CAD build for the part. Positions are in the model's coordinates, mm. A direction names the side the tool comes from. Give positions to 0.01 mm unless a question says otherwise; leave off trailing zeros. Write each loop counter-clockwise with the first axis right and the second up, starting at its lowest first coordinate (ties: lowest second). Pieces come first, ordered by that corner, then holes. Notation, with made-up numbers: (25.25, 55) - (73.25, 55) arc R21 ccw to (73.25, 62) - close; hole circle Ø5 at (51, 0.5). An arc over 180 degrees is marked (long way). Answer as a JSON object with one key per item and string values.
from build123d import *

# Parameters (mm, degrees)
BOSS_EXTRUDE1_DEPTH = 50.8
SKETCH2_W           = 11.43
SKETCH2_H           = 24.13
BOSS_EXTRUDE2_DEPTH = 25.4
FILLET3_R           = 2.54
SKETCH3_R           = 3.175
CUT_EXTRUDE1_DEPTH  = 199.372898559
SKETCH4_W           = 25.146
SKETCH4_H           = 13.208
SKETCH4_W_2         = 25.908
SKETCH4_H_2         = 8.89
CUT_EXTRUDE2_DEPTH  = 25.4
CHAMFER1_SIZE       = 8.89
SKETCH5_R           = 3.175
CUT_EXTRUDE3_DEPTH  = 202.317710741
SKETCH7_W           = 50.8
SKETCH7_H           = 50.8
BOSS_EXTRUDE4_DEPTH = 6.35
FILLET4_R           = 12.7


with BuildPart() as part:
    # Sketch1 → Boss-Extrude1 (new body)
    with BuildSketch(Plane(origin=(0, 0, 0), x_dir=(1, 0, 0), z_dir=(0, 1, 0))):
        Polygon((-59.171267606, -17.601126761), (-59.171267606, 185.598873239), (42.428732394, 185.598873239), (42.428732394, -17.601126761), (17.028732394, -17.601126761), (17.028732394, 160.198873239), (-33.771267606, 160.198873239), (-33.771267606, -17.601126761), align=None)
    extrude(amount=BOSS_EXTRUDE1_DEPTH)

    # Sketch2 → Boss-Extrude2 (add)
    with BuildSketch(Plane.XY.offset(17.601126761)):
        with Locations((-46.471267606, 25.4)):
            Rectangle(SKETCH2_W, SKETCH2_H)
        with Locations((29.728732394, 25.4)):
            Rectangle(SKETCH2_W, SKETCH2_H)
    extrude(amount=BOSS_EXTRUDE2_DEPTH)

    # Fillet3
    fillet3_edges = [part.edges().sort_by_distance(p)[0] for p in [
        (-46.471267606, 37.465, 17.601126761),
        (-46.471267606, 13.335, 17.601126761),
        (29.728732394, 37.465, 17.601126761),
        (29.728732394, 13.335, 17.601126761),
    ]]
    fillet(fillet3_edges, radius=FILLET3_R)

    # Sketch3 → Cut-Extrude1 (cut, through all)
    with BuildSketch(Plane(origin=(0, 37.465, 0), x_dir=(1, 0, 0), z_dir=(0, 1, 0))):
        with Locations(Location((-47.106267606, -30.301126761, 0), (0, 0, 270))):
            Circle(SKETCH3_R)
        with Locations(Location((29.093732394, -30.301126761, 0), (0, 0, 270))):
            Circle(SKETCH3_R)
    extrude(amount=-CUT_EXTRUDE1_DEPTH, mode=Mode.SUBTRACT)

    # Sketch4 → Cut-Extrude2 (cut)
    with BuildSketch(Plane(origin=(0, 0, -185.598873239), x_dir=(-1, 0, 0), z_dir=(0, 0, -1))):
        with Locations((-17.155732394, 25.4)):
            Rectangle(SKETCH4_W, SKETCH4_H)
        with Locations((8.371267606, 25.4)):
            Rectangle(SKETCH4_W_2, SKETCH4_H)
        with Locations((8.371267606, 36.449)):
            Rectangle(SKETCH4_W_2, SKETCH4_H_2)
        with Locations((33.898267606, 25.4)):
            Rectangle(SKETCH4_W, SKETCH4_H)
        with Locations((8.371267606, 14.351)):
            Rectangle(SKETCH4_W_2, SKETCH4_H_2)
    extrude(amount=-CUT_EXTRUDE2_DEPTH, mode=Mode.SUBTRACT)

    # Chamfer1
    chamfer1_edges = [part.edges().sort_by_distance(p)[0] for p in [
        (-21.325267606, 32.004, -172.898873239),
        (-21.325267606, 18.796, -172.898873239),
        (4.582732394, 18.796, -172.898873239),
        (4.582732394, 32.004, -172.898873239),
    ]]
    chamfer(chamfer1_edges, length=CHAMFER1_SIZE - 0.0001)  # a hair under: the kernel refuses the full size

    # Sketch5 → Cut-Extrude3 (cut, through all)
    with BuildSketch(Plane.XZ):
        with Locations(Location((-8.371267606, -172.898873239, 0), (0, 0, 270))):
            Circle(SKETCH5_R)
    extrude(amount=-CUT_EXTRUDE3_DEPTH, mode=Mode.SUBTRACT)

    # Sketch7 → Boss-Extrude4 (add)
    with BuildSketch(Plane.XY.offset(-160.198873239)):
        with Locations((-8.371267606, 25.4)):
            Rectangle(SKETCH7_W, SKETCH7_H)
    extrude(amount=BOSS_EXTRUDE4_DEPTH)

    # Fillet4
    fillet4_edges = [part.edges().sort_by_distance(p)[0] for p in [
        (-33.771267606, 25.4, -153.848873239),
        (17.028732394, 25.4, -153.848873239),
    ]]
    fillet(fillet4_edges, radius=FILLET4_R)


solid = part.part
Item 1: Mould opens along X. For faces 4 (the flat face through (-59.171, 25, -83)), 5 (the flat face through (-9, 26, -160.199)), 6 (the flat face through (35.444, 25, 30)), 7 (the flat face through (-43, 50.8, -108)) say: +X half, -X half, draft (parallel to the pull), parting line (faces both ways), or undercut.
Entries:
{"face 4": "-X half", "face 5": "undercut", "face 6": "+X half", "face 7": "draft"}
Item 2: Flat gauge pins, fed straight in: P1, Ø7.5, axis at y = 23.5, z = 26, coming from the -X side; P2, Ø5.5, axis at x = 30.5, z = 28, coming from the +Y side (3 decimals); P3, Ø1.5, axis at x = 9, y = 27, coming from the +Z side. Where does each tip first touch, or does it go through?
Entries:
{"P1": "x = -52.19", "P2": "y = 37.465", "P3": "z = -152.63"}
Item 3: Cut at D-D (y = 45.5). Give the cut face in (x, z) (3 decimals).
Entries:
{"outline": "(-59.171, -185.599) - (42.429, -185.599) - (42.429, 17.601) - (17.029, 17.601) - (17.029, -141.149) arc R12.7 cw to (4.329, -153.849) - (-21.071, -153.849) arc R12.7 cw to (-33.771, -141.149) - (-33.771, 17.601) - (-59.171, 17.601) - close; hole circle Ø6.35 at (-8.371, -172.899)"}
Item 4: Cut at C-C (x = -38). Give the cut face in (y, z), and give its area (3 significant figures).
Entries:
{"outline": "(0, -185.6) - (18.8, -185.6) - (18.8, -160.2) - (32, -160.2) - (32, -185.6) - (50.8, -185.6) - (50.8, 17.6) - (0, 17.6) - close", "area": "9,990 mm2"}
Item 5: Cut at A-A (z = -48.5). Give the cut face in (x, y), and give its area (3 significant figures).
Entries:
{"outline": "(-59.17, 0) - (-33.77, 0) - (-33.77, 50.8) - (-59.17, 50.8) - close; (17.03, 0) - (42.43, 0) - (42.43, 50.8) - (17.03, 50.8) - close", "area": "2,580 mm2"}
Item 6: Cut at B-B (y = 35). Give the cut face in (x, z) (3 decimals), and give its area (3 significant figures).
Entries:
{"outline": "(-59.171, -185.599) - (-27.219, -185.599) - (-27.219, -160.199) - (10.477, -160.199) - (10.477, -185.599) - (42.429, -185.599) - (42.429, 17.601) - (35.444, 17.601) - (35.444, 43.001) - (24.014, 43.001) - (24.014, 17.601) - (17.029, 17.601) - (17.029, -141.149) arc R12.7 cw to (4.329, -153.849) - (-21.071, -153.849) arc R12.7 cw to (-33.771, -141.149) - (-33.771, 17.601) - (-40.756, 17.601) - (-40.756, 43.001) - (-52.186, 43.001) - (-52.186, 17.601) - (-59.171, 17.601) - close; hole circle Ø6.35 at (-47.106, 30.301); hole circle Ø6.35 at (29.094, 30.301)", "area": "11,600 mm2"}
Item 7: Which spindle directions (+Z, -Z, +X, -X, +Y, -Y) get a long thin tool onto all of the face, cutting with end or side? Do faces 1 (the flat face through (36, 25, 17.601)), 2 (the flat face through (30, 13.335, 34)), 3 (the flat face through (22, 18.796, -173)). Say none if no direction does.
Entries:
{"face 1": "+Z", "face 2": "+Z, +X, -X, -Y", "face 3": "-Z"}
Item 8: Probe line 1 (X direction, y = 19, z = -62); line 2 (Y direction, x = -2, z = -161.5); line 3 (Z direction, x = 31, y = 7.5). List the from-to ranges inside material, lowest first. Write a range as from..to.
Entries:
{"line 1": "-59.17..-33.77, 17.03..42.43", "line 2": "0..9.91, 40.89..50.8", "line 3": "-185.6..17.6"}
